For this review, take the finished solid that the model builds, in its own axes (mm). A direction names the side the tool comes from. Round coordinates to 2 decimals unless told otherwise and drop trailing zeros. Write each loop counter-clockwise with the first axis right and the second up, starting at its lowest first coordinate (ties: lowest second). Pieces come first, ordered by that corner, then holes. Notation, with made-up numbers: (-34.75, 43) -> (-22.75, 43) arc R13 cw to (-22.75, 65) -> close; hole circle Ø5 at (8, 26). An arc over 180 degrees is marked (long way). Answer in a Markdown table with one row per item.
from build123d import *

# Parameters (mm, degrees)
F1_DEPTH = 48.26
F3_DEPTH = 18.288
F5_DEPTH = 28.448
F7_DEPTH = 11.176
F8_R     = 6.35
F9_DEPTH = 35.56


with BuildPart() as f1:
    # F0 (on Top) → F1 (new body)
    with BuildSketch(Plane.XY):
        Polygon((-28.448, 0), (0, 0), (0, 30.48), (0, 60.96), (-28.448, 60.96), (-28.448, 48.26), (-18.288, 48.26), (-18.288, 43.18), (-18.288, 30.48), (-18.288, 17.78), (-18.288, 12.7), (-28.448, 12.7), align=None)
    extrude(amount=F1_DEPTH)

    # F2 (on face) → F3 (cut, through all)
    with BuildSketch(Plane.YZ):
        Polygon((17.78, 38.1), (30.48, 38.1), (43.18, 38.1), (43.18, 48.26), (30.48, 48.26), (17.78, 48.26), align=None)
    extrude(amount=-F3_DEPTH, mode=Mode.SUBTRACT)

    # F4 (on Top) → F5 (join)
    with BuildSketch(Plane.XY):
        Polygon((0, 30.48), (0, 12.7), (60.198, 12.7), (90.932, 30.48), (60.198, 48.26), (0, 48.26), align=None)
    extrude(amount=F5_DEPTH)

    # F6 (on face) → F7 (cut)
    with BuildSketch(Plane.XY.offset(28.448)):
        Polygon((74.22266, 20.81344), (90.932, 30.48), (74.22266, 40.14656), align=None)
    extrude(amount=-F7_DEPTH, mode=Mode.SUBTRACT)

    # F8 (on face) → F9 (cut, through all)
    with BuildSketch(Plane.XZ.offset(-12.7)):
        with Locations((35.052, 14.224)):
            Circle(F8_R)
    extrude(amount=-F9_DEPTH, mode=Mode.SUBTRACT)


solid = f1.part
1) Clearance check with flat-ended pins moving along their axes: pin 1 Ø5.5 at (y, z) = (27, 22.5) entering from +X; pin 2 Ø12 at (x, z) = (28, 9) entering from +Y; pin 3 Ø5 at (x, z) = (-24.5, 18.5) entering from -Y; pin 4 Ø2 at (x, y) = (67, 23.5) entering from +Z. State where each tip first meets the part, or that it passes through.
Solved:
| item | result |
|---|---|
| pin 1 | x = 74.22 |
| pin 2 | y = 48.26 |
| pin 3 | y = 0 |
| pin 4 | z = 28.45 |
2) For line 1 (Z direction, x = 34.5, y = 34); line 2 (Z direction, x = 67, y = 41); line 3 (X direction, y = 12, z = 4), list the stretches that pass through material, from the lowest coordinate up. Write a range as [from, to].
Solved:
| item | result |
|---|---|
| line 1 | [0, 7.9], [20.55, 28.45] |
| line 2 | [0, 28.45] |
| line 3 | [-28.45, 0] |
3) Consider section A-A on z = 39.5. State the section outline as (x, y) points, then the cut area to 3 significant figures.
Solved:
| item | result |
|---|---|
| outline | (-28.45, 0) -> (0, 0) -> (0, 17.78) -> (-18.29, 17.78) -> (-18.29, 12.7) -> (-28.45, 12.7) -> close; (-28.45, 48.26) -> (-18.29, 48.26) -> (-18.29, 43.18) -> (0, 43.18) -> (0, 60.96) -> (-28.45, 60.96) -> close |
| area | 908 mm² |
4) Consider section B-B on y = 19. State the section outline as (x, z) points.
Solved:
| item | result |
|---|---|
| outline | (-18.29, 0) -> (71.09, 0) -> (71.09, 28.45) -> (0, 28.45) -> (0, 38.1) -> (-18.29, 38.1) -> close; hole circle Ø12.7 at (35.05, 14.22) |
5) Consider section D-D on z = 22.5. State the section outline as (x, y) points, then the cut area to 3 significant figures.
Solved:
| item | result |
|---|---|
| outline | (-28.45, 0) -> (0, 0) -> (0, 12.7) -> (60.2, 12.7) -> (74.22, 20.81) -> (74.22, 40.15) -> (60.2, 48.26) -> (0, 48.26) -> (0, 60.96) -> (-28.45, 60.96) -> (-28.45, 48.26) -> (-18.29, 48.26) -> (-18.29, 12.7) -> (-28.45, 12.7) -> close |
| area | 3,900 mm² |
6) Consider section C-C on x = -14. State the section outline as (y, z) points.
Solved:
| item | result |
|---|---|
| outline | (0, 0) -> (60.96, 0) -> (60.96, 48.26) -> (43.18, 48.26) -> (43.18, 38.1) -> (17.78, 38.1) -> (17.78, 48.26) -> (0, 48.26) -> close |
7) Mouldability with a two-part tool opening along X and no side actions: class faces 1 (the flat face through (74.223, 31, 23)), 2 (the flat face through (-18.288, 31, 18)), 3 (the cylindrical face through (41.11, 30.23, 16.13)) as pulls with the +X half, pulls with the -X half, needs draft (parallel to the pull), parting line crosses it, or undercut.
Solved:
| item | result |
|---|---|
| face 1 | pulls with the +X half |
| face 2 | pulls with the -X half |
| face 3 | undercut |
8) For faces 4 (the flat face through (37, 31, 28.448)), 5 (the flat face through (-23, 12.7, 24)), 6 (the flat face through (31, 48.26, 20)), 7 (the flat face through (-9, 17.78, 43)), list the 3-axis set-ups (+Z, -Z, +X, -X, +Y, -Y) from which the entire face can be reached by the end or side of a thin tool; tool diameter is ignored.
Solved:
| item | result |
|---|---|
| face 4 | +Z, +X, +Y, -Y |
| face 5 | +Z, -Z, -X |
| face 6 | +Z, -Z, +X, +Y |
| face 7 | +Z, +X, -X |
